Input: part model. Units: mm. Frame: model coordinates. Face numbers are marked on the shaded views. A direction names the side the tool comes from. Coordinates: 2 decimals unless noted, no trailing zeros. Loops run counter-clockwise (first coordinate to the right, second up) from the corner with the lowest first, then second, coordinate; pieces in that order, holes last. Notation, with made-up numbers: (-7, -3.75) -> (34, -3.75) arc R8 cw to (34, 5.25) -> close; hole circle Ø2 at (23, -5). An arc over 180 degrees is marked (long way). Put each result on its own line as item: value. Start each with the question number.
1) Material intervals for L1, parallel to Z at x = 15, y = 4.5; L2, parallel to Y at x = 6.75, z = -39.5; L3, parallel to Z at x = 23.25, y = 70.5, sorted ascending.
2) Cut plane D-D (x = 26). Return the cut outline in (y, z).
3) Cut plane A-A (y = 105). Return the cut outline in (x, z), plus the area to 3 significant figures.
4) Contact query for flat-ended pins moving along their axis: P1, Ø9, axis at x = 21.5, z = -26.5, coming from the +Y side; P2, Ø1.5, axis at x = 13.5, y = 14.5, coming from the +Z side; P3, Ø1.5, axis at x = 21.5, y = 120.5, coming from the -Z side. Output: stop coordinate, or through.
5) Cut plane B-B (x = 15). Return the cut outline in (y, z).
6) Cut plane C-C (z = -45). Return the cut outline in (x, y).
7) Set-up query: the marked faces 1 and 2. Return all of +Z, -Z, +X, -X, +Y, -Y with unobstructed straight access to the full face (end or side cutting, diameter ignored); none if empty.
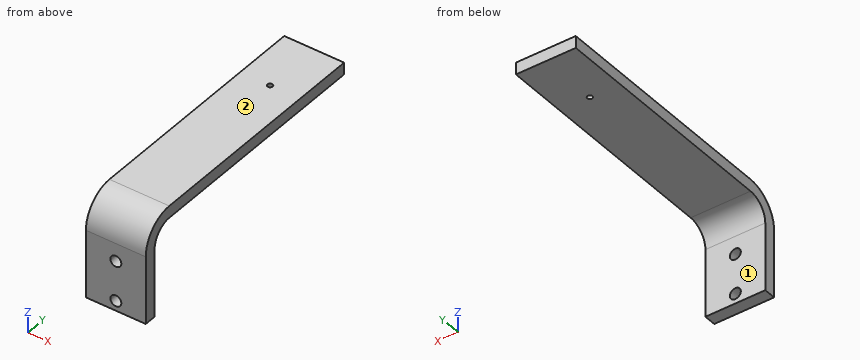
from build123d import *

# Parameters (mm, degrees)
BOSS_EXTRUDE1_DEPTH   = 30
FILLET1_R             = 10
FILLET2_R             = 16
M5_CLEARANCE_HOLE1_D  = 5.5
F_5_40_TAPPED_HOLE1_D = 2.5781


with BuildPart() as part:
    # Sketch1 → Boss-Extrude1 (new body)
    with BuildSketch(Plane(origin=(0, 0, 0), x_dir=(0, 0, -1), z_dir=(1, 0, 0))):
        Polygon((0, 0), (50, 0), (50, 6), (6, 6), (6, 135), (0, 135), align=None)
    extrude(amount=BOSS_EXTRUDE1_DEPTH)

    # Fillet1
    fillet1_edges = [part.edges().sort_by_distance(p)[0] for p in [
        (15, 6, -6),
    ]]
    fillet(fillet1_edges, radius=FILLET1_R)

    # Fillet2
    fillet2_edges = [part.edges().sort_by_distance(p)[0] for p in [
        (15, 0, 0),
    ]]
    fillet(fillet2_edges, radius=FILLET2_R)

    # M5 Clearance Hole1 (through all)
    with Locations(Plane(origin=(0, 6, 0), x_dir=(1, 0, 0), z_dir=(0, 1, 0))):
        with Locations((15, 45), (15, 25)):
            Hole(M5_CLEARANCE_HOLE1_D / 2)

    # #5-40 Tapped Hole1 (through all)
    with Locations(Plane.XY):
        with Locations((15, 105)):
            Hole(F_5_40_TAPPED_HOLE1_D / 2)


solid = part.part
Results found:
1. L1: z = -50 to -47.75, -42.25 to -27.75, -22.25 to -4.88
1. L2: y = 0 to 6
1. L3: z = -6 to 0
2. outline: (0, -50) -> (6, -50) -> (6, -16) arc R10 cw to (16, -6) -> (135, -6) -> (135, 0) -> (16, 0) arc R16 ccw to (0, -16) -> close
3. outline: (0, -6) -> (13.71, -6) -> (13.71, 0) -> (0, 0) -> close; (16.29, -6) -> (30, -6) -> (30, 0) -> (16.29, 0) -> close
3. area: 165 mm2
4. P1: stops at y = 6
4. P2: stops at z = -0.02
4. P3: stops at z = -6
5. outline: (0, -50) -> (6, -50) -> (6, -47.75) -> (0, -47.75) -> close; (0, -42.25) -> (6, -42.25) -> (6, -27.75) -> (0, -27.75) -> close; (0, -22.25) -> (6, -22.25) -> (6, -16) arc R10 cw to (16, -6) -> (103.71, -6) -> (103.71, 0) -> (16, 0) arc R16 ccw to (0, -16) -> close; (106.29, -6) -> (135, -6) -> (135, 0) -> (106.29, 0) -> close
6. outline: (0, 0) -> (12.25, 0) -> (12.25, 6) -> (0, 6) -> close; (17.75, 0) -> (30, 0) -> (30, 6) -> (17.75, 6) -> close
7. face 1: -Z, +X, -X, +Y
7. face 2: +Z, +X, -X, +Y, -Y
